Design review of the part built by this model. Coordinates are the model's own, in mm. Face numbers are marked on the shaded views. Coordinates: 2 decimals unless noted, no trailing zeros. Order: outer loops, then holes, each group sorted by start corner. A loop starts at its lowest first (then second) coordinate and runs counter-clockwise, first axis right, second up. Notation, with made-up numbers: M -27.75,10 L 3.25,10 A22 ccw 3.25,16 Z; hole C 72,48 d4. An arc over 180 degrees is marked long. Answer as a JSON object with one key per item and string values.
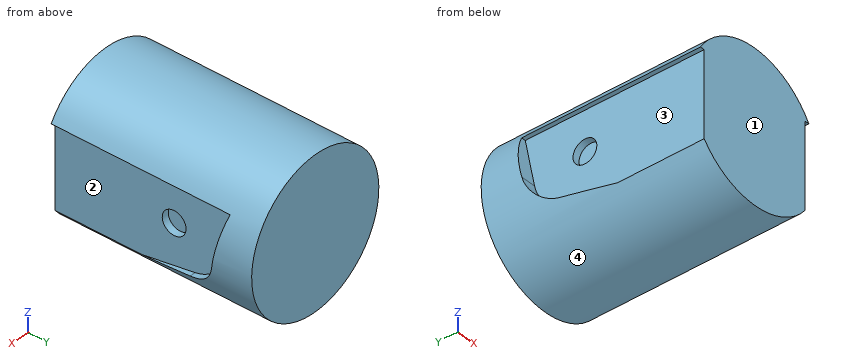
from build123d import *

# Parameters (mm, degrees)
SKETCH_1_R          = 31.5
EXTRUDE_1_DEPTH     = 88
CUT_EXTRUDE_1_DEPTH = 6.5
SKETCH_3_R          = 5
CUT_EXTRUDE_2_DEPTH = 3


with BuildPart() as part:
    # 草图1 → 凸台-拉伸1 (new body)
    with BuildSketch(Plane(origin=(0, 0, 0), x_dir=(1, 0, 0), z_dir=(0, 1, 0))):
        with Locations(Location((0, 0, 0), (0, 0, 270))):
            Circle(SKETCH_1_R)
    extrude(amount=EXTRUDE_1_DEPTH)

    # 草图2 → 切除-拉伸1 (cut)
    with BuildSketch(Plane(origin=(31.5, 0, 0), x_dir=(0, 0, -1), z_dir=(1, 0, 0))):
        with BuildLine():
            Line((-16.5, 75), (3.625312861, 71.114880191))
            ThreePointArc((3.625312861, 71.114880191), (11.558802441, 66.820544019), (15.59440661, 58.752367083))
            Line((15.59440661, 58.752367083), (24.977312136, 0))
            Line((24.977312136, 0), (-16.5, 0))
            Line((-16.5, 0), (-16.5, 75))
        make_face()
    cut_extrude_1 = extrude(amount=-CUT_EXTRUDE_1_DEPTH, mode=Mode.SUBTRACT)

    # 镜向1: 切除-拉伸1 across plane
    add(cut_extrude_1.mirror(Plane(origin=(0, 0, 0), x_dir=(0, 0, 1), z_dir=(1, 0, 0))), mode=Mode.SUBTRACT)

    # 草图3 → 切除-拉伸2 (cut)
    with BuildSketch(Plane(origin=(25, 0, 0), x_dir=(0, 0, -1), z_dir=(1, 0, 0))):
        with Locations((0, 50)):
            Circle(SKETCH_3_R)
    cut_extrude_2 = extrude(amount=-CUT_EXTRUDE_2_DEPTH, mode=Mode.SUBTRACT)

    # 镜向2: 切除-拉伸2 across plane
    add(cut_extrude_2.mirror(Plane(origin=(0, 0, 0), x_dir=(0, 0, 1), z_dir=(1, 0, 0))), mode=Mode.SUBTRACT)


solid = part.part
1) Add section D-D (z = 0). State the section outline as (x, y) points, and give its area (3 significant figures).
Taken from the geometry:
{"outline": "M -31.5,71.81 L -25,71.81 L -25,55 L -22,55 L -22,45 L -25,45 L -25,0 L 25,0 L 25,45 L 22,45 L 22,55 L 25,55 L 25,71.81 L 31.5,71.81 L 31.5,88 L -31.5,88 Z", "area": "4,550 mm2"}
2) To check wall thickness, follow L1, parallel to Y at x = -23.2, z = 0; L2, parallel to X at y = 53.5, z = 10; L3, parallel to Z at x = -26, y = 53. State the ranges of each line that lie inside material, in increasing order.
Taken from the geometry:
{"L1": "y = 0 to 45, 55 to 88", "L2": "x = -25 to 25", "L3": "z = -17.78 to -16.51, 16.5 to 17.78"}
3) Insertion check: pin 1 Ø10.5 at (y, z) = (53, 6) entering from -X; pin 2 Ø1 at (y, z) = (15.5, 21) entering from -X; pin 3 Ø13 at (y, z) = (50, 0) entering from +X. Each pin has a flat end and moves straight along its axis. Give the tip position at first contact, or say it passes through.
Taken from the geometry:
{"pin 1": "stops at x = -25", "pin 2": "stops at x = -23.92", "pin 3": "stops at x = 25"}
4) Add section B-B (z = 15). State the section outline as (x, y) points.
Taken from the geometry:
{"outline": "M -27.7,74.71 L -25,74.71 L -25,0 L 25,0 L 25,74.71 L 27.7,74.71 L 27.7,88 L -27.7,88 Z"}
5) Add section C-C (x = -10.5). State the section outline as (y, z) points, and give its area (3 significant figures).
Taken from the geometry:
{"outline": "M 0,-29.7 L 88,-29.7 L 88,29.7 L 0,29.7 Z", "area": "5,230 mm2"}
6) Mouldability with a two-part tool opening along Z and no side actions: class the marked faces 1, 2, 3 and 4 as released by +Z, released by -Z, zero draft, split by the parting line, or undercut.
Taken from the geometry:
{"face 1": "zero draft", "face 2": "undercut", "face 3": "undercut", "face 4": "split by the parting line"}
7) Add section A-A (y = 21). State the section outline as (x, z) points.
Taken from the geometry:
{"outline": "M -26.83,16.5 L -25,16.5 L -25,-19.16 A31.5 ccw 25,-19.16 L 25,16.5 L 26.83,16.5 A31.5 ccw Z"}
